Read the model definition and answer for the solid it produces. Units are mm, in the model's axes. A direction names the side the tool comes from. Coordinates: 2 decimals unless noted, no trailing zeros. Write each loop counter-clockwise with the first axis right and the second up, starting at its lowest first coordinate (ties: lowest second). Pieces come first, ordered by that corner, then holes. Notation, with made-up numbers: (11.25, 49) -> (41.25, 49) arc R17 cw to (41.25, 72) -> close; hole circle Ø1 at (84.5, -15.75). An arc over 180 degrees is marked (long way). Write item = value, one per line. Start each with the question number.
1) Section B-B (z = 0) is taken. Determine the outline of the cut face in (x, y), plus the area to 4 significant figures.
2) Find the intervals of material crossed by line 1 along Y through (x, z) = (2.5, 9); line 2 along Y through (x, z) = (14.25, -10.75); line 3 along X through (y, z) = (-4.5, 5.5), in increasing order. Write a range as from..to.
3) Section C-C (y = 4.5) is taken. Determine the outline of the cut face in (x, z).
4) Section A-A (y = 0) is taken. Determine the outline of the cut face in (x, z).
5) For a pull along Y with two mould halves and no side action, classify faces 1 (the face through (15, 3, 3)), 2 (the face through (7.4, 11.89, -0.99)), 3 (the face through (7.395, 2.733, -11.612)) as released by +Y, released by -Y, zero draft, split by the parting line, or undercut.
6) Flat-ended cylindrical pins translate along their axes: pin 1 Ø1 at (x, y) = (14, 6.5) entering from -Z; pin 2 Ø0.6 at (x, y) = (14, 7) entering from +Z; pin 3 Ø0.5 at (x, y) = (14, 5.5) entering from +Z; pin 4 Ø4.5 at (y, z) = (-1, -0.5) entering from -X. Find the tip coordinate at first contact, or state that the pin passes through.
7) A tool of negligible diameter and unlimited length cuts with its end or side. For faces 4 (the face through (7.4, 9.04, -7.79)), 5 (the face through (7.4, -11.89, 0.99)), 6 (the face through (7.4, 10.16, -6.18)), from which of +Z, -Z, +X, -X, +Y, -Y can it reach the whole face along a straight path? Write none if from no direction.
from build123d import *

# Parameters (mm, degrees)
BASPROSKE_W         = 15
BASPROSKE_H         = 13.2
TOOTHCUT_DEPTH      = 24.947442452
TEETHCUTS_COUNT     = 20
TEETHCUTS_ANGLE     = 342
BORSKE_R            = 4
BORE_DEPTH          = 50.0000508
BOSS_EXTRUDE1_START = -15
BOSS_EXTRUDE1_DEPTH = 15
SKETCH2_R           = 7.2
SKETCH2_R_2         = 6
CUT_EXTRUDE1_DEPTH  = 0.5
CUT_EXTRUDE2_DEPTH  = 2


with BuildPart() as part:
    # BasProSke → Base-Revolve (revolve)
    with BuildSketch(Plane(origin=(0, 0, 0), x_dir=(1, 0, 0), z_dir=(0, 1, 0)), mode=Mode.PRIVATE) as base_revolve_sk:
        with Locations((7.5, 6.6)):
            Rectangle(BASPROSKE_W, BASPROSKE_H)
    revolve(base_revolve_sk.sketch.rotate(Axis((-10, 0, 0), (1, 0, 0)), 180), axis=Axis((-10, 0, 0), (1, 0, 0)))

    # TooCutSke → ToothCut (cut, through all)
    with BuildSketch(Plane(origin=(0, 0, 0), x_dir=(0, 0, -1), z_dir=(1, 0, 0))):
        with BuildLine():
            ThreePointArc((0.599012827, 10.48189795), (0, 10.499), (-0.599012827, 10.48189795))
            ThreePointArc((-0.599012827, 10.48189795), (-0.986906343, 11.883983562), (-1.777012823, 13.105473306))
            ThreePointArc((-1.777012823, 13.105473306), (0, 13.2254), (1.777012823, 13.105473306))
            ThreePointArc((1.777012823, 13.105473306), (0.986906343, 11.883983562), (0.599012827, 10.48189795))
        make_face()
    toothcut = extrude(amount=TOOTHCUT_DEPTH, mode=Mode.SUBTRACT)

    # TeethCuts: ToothCut ×20 about axis
    teethcuts_axis = Axis((-10, 0, 0), (1, 0, 0))
    for i in range(1, TEETHCUTS_COUNT):
        add(toothcut.rotate(teethcuts_axis, i * TEETHCUTS_ANGLE / (TEETHCUTS_COUNT - 1)), mode=Mode.SUBTRACT)

    # BorSke → Bore (cut, symmetric)
    with BuildSketch(Plane(origin=(0, 0, 0), x_dir=(0, 0, -1), z_dir=(1, 0, 0))):
        with Locations(Location((0, 0, 0), (0, 0, 180))):
            Circle(BORSKE_R)
    extrude(amount=BORE_DEPTH, both=True, mode=Mode.SUBTRACT)

    # Sketch1 → Boss-Extrude1 (add)
    with BuildSketch(Plane.ZY.offset(BOSS_EXTRUDE1_START)):
        with BuildLine():
            Line((3.067450983, 2.567244528), (-2.628080047, 3.015492541))
            ThreePointArc((-2.628080047, 3.015492541), (0.313836383, 3.987669335), (3.067450983, 2.567244528))
        make_face()
    extrude(amount=BOSS_EXTRUDE1_DEPTH)

    # Sketch2 → Cut-Extrude1 (cut)
    with BuildSketch(Plane.ZY):
        Circle(SKETCH2_R)
        Circle(SKETCH2_R_2, mode=Mode.SUBTRACT)
    extrude(amount=-CUT_EXTRUDE1_DEPTH, mode=Mode.SUBTRACT)

    # Sketch3 → Cut-Extrude2 (cut)
    with BuildSketch(Plane(origin=(15, 0, 0), x_dir=(0, 0, -1), z_dir=(1, 0, 0))):
        Polygon((-0.996764222, 8.228081038), (-0.426892427, 8.228081038), (-0.426892427, 5.622952833), (0.468620394, 5.622952833), (0.468620394, 5.053081038), (-0.996764222, 5.053081038), align=None)
    extrude(amount=-CUT_EXTRUDE2_DEPTH, mode=Mode.SUBTRACT)


solid = part.part
Answer key:
q1.outline = (0, -10.5) -> (15, -10.5) -> (15, -4) -> (0, -4) -> (0, -6) -> (0.5, -6) -> (0.5, -7.2) -> (0, -7.2) -> close; (0, 2.81) -> (15, 2.81) -> (15, 5.05) -> (13, 5.05) -> (13, 5.62) -> (15, 5.62) -> (15, 10.5) -> (0, 10.5) -> (0, 7.2) -> (0.5, 7.2) -> (0.5, 6) -> (0, 6) -> close
q1.area = 210.5 mm^2
q2.line_1 = -9.52..-7.72, -5.77..5.77, 7.72..9.52
q2.line_2 = -6.27..-4.4, -2.75..-0.64, 0.64..2.75, 4.4..6.27
q2.line_3 = 0.5..15
q3.outline = (0, -10.87) -> (15, -10.87) -> (15, 10.87) -> (0, 10.87) -> (0, 5.62) -> (0.5, 5.62) -> (0.5, 3.97) -> (0, 3.97) -> (0, -3.97) -> (0.5, -3.97) -> (0.5, -5.62) -> (0, -5.62) -> close
q4.outline = (0, -10.5) -> (15, -10.5) -> (15, -4) -> (0, -4) -> (0, -6) -> (0.5, -6) -> (0.5, -7.2) -> (0, -7.2) -> close; (0, 4) -> (15, 4) -> (15, 10.5) -> (0, 10.5) -> (0, 7.2) -> (0.5, 7.2) -> (0.5, 6) -> (0, 6) -> close
q5.face_1 = zero draft
q5.face_2 = released by +Y
q5.face_3 = undercut
q6.pin_1 = -11.76
q6.pin_2 = 8.72
q6.pin_3 = 11.9
q6.pin_4 = through
q7.face_4 = +X, -X, +Y
q7.face_5 = +X, -X, -Y
q7.face_6 = +X, -X
